Build history of the part. All positions in model axes, mm. Face numbers are marked on the shaded views. A direction names the side the tool comes from. Give positions to 0.01 mm unless a question says otherwise; leave off trailing zeros. Write each loop counter-clockwise with the first axis right and the second up, starting at its lowest first coordinate (ties: lowest second). Pieces come first, ordered by that corner, then holes. Notation, with made-up numbers: (-11.75, 17.5) - (46.25, 17.5) arc R34 cw to (46.25, 52.5) - close; hole circle Ø11 at (34.25, -14.5). An arc over 180 degrees is marked (long way). Use one line per item in the form item = value. Start each with the question number.
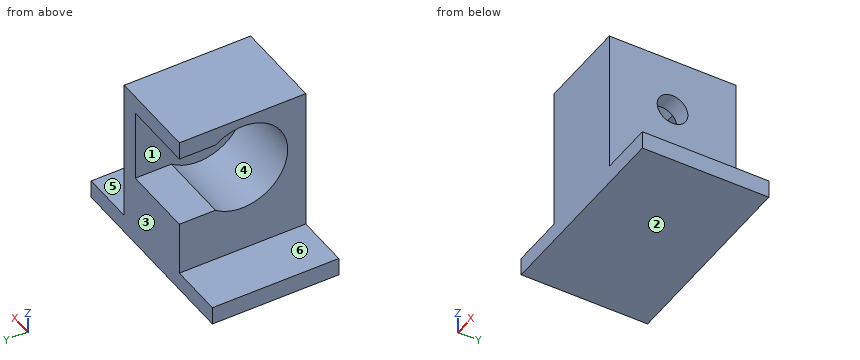
from build123d import *

# Parameters (mm, degrees)
F0_W      = 25
F0_H      = 35
F1_DEPTH  = 45
F2_R      = 12.5
F3_DEPTH  = 20
F4_R      = 4.25
F5_DEPTH  = 25
F6_W      = 35
F6_H      = 5
F7_DEPTH  = 15
F8_W      = 35
F8_H      = 5
F9_DEPTH  = 40
F10_W     = 17.5
F10_H     = 20
F11_DEPTH = 20


with BuildPart() as f1:
    # F0 (on Top) → F1 (new body)
    with BuildSketch(Plane.XY):
        with Locations((12.5, 17.5)):
            Rectangle(F0_W, F0_H)
    extrude(amount=F1_DEPTH)

    # F2 (on Right) → F3 (cut)
    with BuildSketch(Plane.YZ):
        with Locations((17.5, 30)):
            Circle(F2_R)
    extrude(amount=F3_DEPTH, mode=Mode.SUBTRACT)

    # F4 (on Right) → F5 (cut)
    with BuildSketch(Plane.YZ):
        with Locations((17.5, 30)):
            Circle(F4_R)
    extrude(amount=F5_DEPTH, mode=Mode.SUBTRACT)

    # F6 (on Right) → F7 (join)
    with BuildSketch(Plane.YZ):
        with Locations((17.5, 2.5)):
            Rectangle(F6_W, F6_H)
    extrude(amount=-F7_DEPTH)

    # F8 (on Right) → F9 (join)
    with BuildSketch(Plane.YZ):
        with Locations((17.5, 2.5)):
            Rectangle(F8_W, F8_H)
    extrude(amount=F9_DEPTH)

    # F10 (on Right) → F11 (cut)
    with BuildSketch(Plane.YZ):
        with Locations((26.25, 30)):
            Rectangle(F10_W, F10_H)
    extrude(amount=F11_DEPTH, mode=Mode.SUBTRACT)


solid = f1.part
(1) Wall check: line 1 (Y direction, x = 22.75, z = 30); line 2 (Z direction, x = 9, y = 31.5); line 3 (Z direction, x = 6.5, y = 17.5). Give the ranges that are in metal, low to high. Write a range as from..to.
(2) Cut at C-C, the plane y = 32. Give the cut face in (x, z), then the cut area to 3 significant figures.
(3) Which spindle directions (+Z, -Z, +X, -X, +Y, -Y) get a long thin tool onto all of the face, cutting with end or side? Do the marked faces 4, 5 and 6. Say none if no direction does.
(4) Cut at B-B, the plane y = 17.5. Give the cut face in (x, z).
(5) Cut at A-A, the plane z = 30. Give the cut face in (x, y).
(6) Pin check, flat tips, straight feed: pin 1 Ø10 at (y, z) = (9, 12.5) entering from -X; pin 2 Ø12.5 at (y, z) = (14, 26.5) entering from -X; pin 3 Ø2 at (x, z) = (9.5, 21.5) entering from +Y. Stop position of each tip, or through.
(7) Two-plate mould, pull along Z, no slides. Class the marked faces 1, 2 and 3: +Z half, -Z half, draft (parallel to the pull), parting line (faces both ways), or undercut.
(8) Cut at D-D, the plane x = 7.5. Give the cut face in (y, z), then the cut area to 3 significant figures.
Solution:
q1.line_1 = 0..13.25, 21.75..35
q1.line_2 = 0..20, 40..45
q1.line_3 = 0..17.5, 42.5..45
q2.outline = (-15, 0) - (40, 0) - (40, 5) - (25, 5) - (25, 45) - (0, 45) - (0, 40) - (20, 40) - (20, 20) - (0, 20) - (0, 5) - (-15, 5) - close
q2.area = 875 mm2
q3.face_4 = -X
q3.face_5 = +Z, +X, +Y, -Y
q3.face_6 = +Z, -X, +Y, -Y
q4.outline = (-15, 0) - (40, 0) - (40, 5) - (25, 5) - (25, 25.75) - (20, 25.75) - (20, 17.5) - (0, 17.5) - (0, 5) - (-15, 5) - close; (0, 42.5) - (20, 42.5) - (20, 34.25) - (25, 34.25) - (25, 45) - (0, 45) - close
q5.outline = (0, 0) - (25, 0) - (25, 13.25) - (20, 13.25) - (20, 5) - (0, 5) - close; (20, 21.75) - (25, 21.75) - (25, 35) - (20, 35) - close
q6.pin_1 = 0
q6.pin_2 = 20
q6.pin_3 = 9.38
q7.face_1 = undercut
q7.face_2 = -Z half
q7.face_3 = draft
q8.outline = (0, 0) - (35, 0) - (35, 20) - (25, 20) arc R12.5 cw (long way) to (25, 40) - (35, 40) - (35, 45) - (0, 45) - close
q8.area = 954 mm2
